The listing builds one solid part. Answer for the finished solid, in the listing's coordinates (mm). Give positions to 0.01 mm unless a question says otherwise; leave off trailing zeros. Write each loop counter-clockwise with the first axis right and the second up, starting at its lowest first coordinate (ties: lowest second). Pieces come first, ordered by that corner, then holes.
Autodesk Inventor part; units mm, degrees
ref_plane "YZ Plane" through (0, 0, 0) normal (1, 0, 0) x (0, 1, 0)
ref_plane "XZ Plane" through (0, 0, 0) normal (0, 1, 0) x (-1, 0, 0)
ref_plane "XY Plane" through (0, 0, 0) normal (0, 0, 1) x (1, 0, 0)
sketch "Sketch4" plane through (0, 0, 0) normal (1, 0, 0) x (0, 1, 0)
  line L0 (0, 0) -> (0, -26.0096)
  line L1 (0, 0) -> (33.46, 0)
  line L2 (33.46, 0) -> (33.46, -26.0096)
  line L3 (33.46, -26.0096) -> (0, -26.0096)
  line L4 (35.286, -25.908) -> (35.1766, -0.1801)
  arc A0 (35.286, -25.908) -> (35.2799, -24.4856) centre (35.283, -25.1968) ccw
  arc A1 (35.2795, -24.384) -> (35.2735, -22.9616) centre (35.2765, -23.6728) ccw
  arc A2 (35.273, -22.86) -> (35.267, -21.4376) centre (35.27, -22.1488) ccw
  arc A3 (35.2665, -21.336) -> (35.2605, -19.9137) centre (35.2635, -20.6248) ccw
  arc A4 (35.2601, -19.8121) -> (35.254, -18.3897) centre (35.257, -19.1009) ccw
  arc A5 (35.2536, -18.2881) -> (35.2475, -16.8657) centre (35.2506, -17.5769) ccw
  arc A6 (35.2471, -16.7641) -> (35.2411, -15.3417) centre (35.2441, -16.0529) ccw
  arc A7 (35.2406, -15.2401) -> (35.2346, -13.8177) centre (35.2376, -14.5289) ccw
  arc A8 (35.2342, -13.7161) -> (35.2281, -12.2937) centre (35.2311, -13.0049) ccw
  arc A9 (35.2277, -12.1921) -> (35.2216, -10.7697) centre (35.2247, -11.4809) ccw
  arc A10 (35.2212, -10.6681) -> (35.2152, -9.2458) centre (35.2182, -9.9569) ccw
  arc A11 (35.2147, -9.1442) -> (35.2087, -7.7218) centre (35.2117, -8.433) ccw
  arc A12 (35.2083, -7.6202) -> (35.2022, -6.1978) centre (35.2052, -6.909) ccw
  arc A13 (35.2018, -6.0962) -> (35.1957, -4.6738) centre (35.1988, -5.385) ccw
  arc A14 (35.1953, -4.5722) -> (35.1893, -3.1498) centre (35.1923, -3.861) ccw
  arc A15 (35.1888, -3.0482) -> (35.1828, -1.6258) centre (35.1858, -2.337) ccw
  arc A16 (35.1824, -1.5242) -> (35.1763, -0.1018) centre (35.1793, -0.813) ccw
  line L5 (35.1763, -0.1018) -> (33.46, -0.1018)
  line L6 (35.286, -25.908) -> (33.46, -25.908)
  point P0 (35.2799, -24.4856)
  point P1 (35.2735, -22.9616)
  point P2 (35.267, -21.4376)
  point P3 (35.2605, -19.9137)
  point P4 (35.254, -18.3897)
  point P5 (35.2536, -18.2881)
  point P6 (35.2475, -16.8657)
  point P7 (35.2411, -15.3417)
  point P8 (35.2406, -15.2401)
  point P9 (35.2346, -13.8177)
  point P10 (35.2342, -13.7161)
  point P11 (35.2281, -12.2937)
  point P12 (35.2277, -12.1921)
  point P13 (35.2216, -10.7697)
  point P14 (35.2152, -9.2458)
  point P15 (35.2087, -7.7218)
  point P16 (35.2083, -7.6202)
  point P17 (35.2022, -6.1978)
  point P18 (35.2018, -6.0962)
  point P19 (35.1957, -4.6738)
  point P20 (35.1953, -4.5722)
  point P21 (35.1893, -3.1498)
  point P22 (35.1888, -3.0482)
  point P23 (35.1828, -1.6258)
  point P24 (35.1824, -1.5242)
  dimension "d12" = 26.0096
  dimension "d13" = 33.46
  dimension "d14" = 1.8288
  dimension "d18" = 1.524
  dimension "d25" = 0.7112
  dimension "d26" = 0.243
  dimension "d27" = 0.1016
  dimension "d28" = 0
revolve "Revolution1" add sketch "Sketch4" angle 360 about axis through (0, 0, 0) along (0, 0, -1) contours L1 L2 L3 L0
sketch "Sketch5" plane through (0, 0, 0) normal (0, 0, 1) x (1, 0, 0)
  line L0 (19.05, 5.08) -> (19.05, -5.08)
  line L1 (28.575, 10.16) -> (28.575, -10.16)
  line L2 (28.575, 10.16) -> (19.05, 5.08)
  line L3 (19.05, -5.08) -> (28.575, -10.16)
  line L4 (5.4887, 29.8267) -> (5.1256, 19.0378)
  line L5 (5.4887, 29.8267) -> (23.0863, 19.6667)
  line L6 (5.1256, 19.0378) -> (13.9244, 13.9578)
  line L7 (13.9244, 13.9578) -> (23.0863, 19.6667)
  line L8 (-23.0863, 19.6667) -> (-13.9244, 13.9578)
  line L9 (-23.0863, 19.6667) -> (-5.4887, 29.8267)
  line L10 (-13.9244, 13.9578) -> (-5.1256, 19.0378)
  line L11 (-5.1256, 19.0378) -> (-5.4887, 29.8267)
  line L12 (-28.575, -10.16) -> (-19.05, -5.08)
  line L13 (-28.575, -10.16) -> (-28.575, 10.16)
  line L14 (-19.05, -5.08) -> (-19.05, 5.08)
  line L15 (-19.05, 5.08) -> (-28.575, 10.16)
  line L16 (-5.4887, -29.8267) -> (-5.1256, -19.0378)
  line L17 (-5.4887, -29.8267) -> (-23.0863, -19.6667)
  line L18 (-5.1256, -19.0378) -> (-13.9244, -13.9578)
  line L19 (-13.9244, -13.9578) -> (-23.0863, -19.6667)
  line L20 (23.0863, -19.6667) -> (13.9244, -13.9578)
  line L21 (23.0863, -19.6667) -> (5.4887, -29.8267)
  line L22 (13.9244, -13.9578) -> (5.1256, -19.0378)
  line L23 (5.1256, -19.0378) -> (5.4887, -29.8267)
  point P0 (0, 0)
  point P1 (19.05, 0)
  point P2 (28.575, 0)
  point P3 (14.2875, 24.7467)
  point P4 (9.525, 16.4978)
  point P5 (-14.2875, 24.7467)
  point P6 (-9.525, 16.4978)
  point P7 (-28.575, 0)
  point P8 (-19.05, 0)
  point P9 (-14.2875, -24.7467)
  point P10 (-9.525, -16.4978)
  point P11 (14.2875, -24.7467)
  point P12 (9.525, -16.4978)
  dimension "d30" = 10.16
  dimension "d31" = 20.32
  dimension "d32" = 0
  dimension "d33" = 19.05
  dimension "d34" = 9.525
  dimension "d35" = 0
  dimension "d38" = 360
extrude "Extrusion3" cut sketch "Sketch5" against normal through all
fillet "Fillet1" radius 2.54 24 edges at (-5.4887, -29.8267, -13.0048) (-5.1256, -19.0378, -13.0048) (-13.9244, -13.9578, -13.0048) (-23.0863, -19.6667, -13.0048) (5.4887, 29.8267, -13.0048) (5.1256, 19.0378, -13.0048) (13.9244, 13.9578, -13.0048) (23.0863, 19.6667, -13.0048) (-28.575, -10.16, -13.0048) (-19.05, -5.08, -13.0048) (-19.05, 5.08, -13.0048) (-28.575, 10.16, -13.0048) (23.0863, -19.6667, -13.0048) (13.9244, -13.9578, -13.0048) (5.1256, -19.0378, -13.0048) (5.4887, -29.8267, -13.0048) (28.575, 10.16, -13.0048) (19.05, 5.08, -13.0048) (19.05, -5.08, -13.0048) (28.575, -10.16, -13.0048) (-23.0863, 19.6667, -13.0048) (-13.9244, 13.9578, -13.0048) (-5.1256, 19.0378, -13.0048) (-5.4887, 29.8267, -13.0048)
sketch "Sketch6" plane through (0, 0, 0) normal (0, 0, 1) x (1, 0, 0)
  circle A0 centre (0, 0) radius 7.1
  circle A1 centre (-9.798, 5.6569) radius 2 construction
  circle A2 centre (5.6569, 9.798) radius 2 construction
  circle A3 centre (9.798, -5.6569) radius 2 construction
  circle A4 centre (-5.6569, -9.798) radius 2 construction
  circle A5 centre (-9.798, 5.6569) radius 2.15
  circle A6 centre (5.6569, 9.798) radius 2.15
  circle A7 centre (9.798, -5.6569) radius 2.15
  circle A8 centre (-5.6569, -9.798) radius 2.15
  dimension "d43" = 14.2
  dimension "d46" = 4.3
  dimension "d47" = 4.3
  dimension "d48" = 4.3
  dimension "d49" = 4.3
extrude "Extrusion4" cut sketch "Sketch6" against normal through all
properties part number "Wheel_Base"
Item 1: Consider probe 1 along X at (y, z) = (2, -21) (3 decimals); probe 2 along X at (y, z) = (1, -13) (3 decimals); probe 3 along X at (y, z) = (-20.5, -20). Determine where each line is inside the solid, lowest interval first.
Conclusion:
probe 1: x = -33.4 to -28.575, -19.05 to -6.812, 6.812 to 19.05, 28.575 to 33.4
probe 2: x = -33.445 to -28.575, -19.05 to -7.029, 7.029 to 19.05, 28.575 to 33.445
probe 3: x = -26.44 to -20.52, -5.18 to 5.18, 20.52 to 26.44
Item 2: A cutting plane is placed at B-B, the plane x = 0. Give the vertices of the cut face in (y, z).
Conclusion:
outline: (-33.46, -26.01) - (-7.1, -26.01) - (-7.1, 0) - (-33.46, 0) - close; (7.1, -26.01) - (33.46, -26.01) - (33.46, 0) - (7.1, 0) - close
Item 3: A cutting plane is placed at C-C, the plane x = 10.5. Give the vertices of the cut face in (y, z), plus the area to 3 significant figures.
Conclusion:
outline: (-31.77, -26.01) - (-26.93, -26.01) - (-26.93, 0) - (-31.77, 0) - close; (-15.93, -26.01) - (-7.69, -26.01) - (-7.69, 0) - (-15.93, 0) - close; (-3.62, -26.01) - (15.93, -26.01) - (15.93, 0) - (-3.62, 0) - close; (26.93, -26.01) - (31.77, -26.01) - (31.77, 0) - (26.93, 0) - close
area: 975 mm2
Item 4: Determine the mould class of faces 1 (the face through (-0.92, 7.04, -12.82)), 2 (the face through (-9.482, -16.523, -12.823)) for opening direction Y: pulls with the +Y half, pulls with the -Y half, needs draft (parallel to the pull), parting line crosses it, or undercut.
Conclusion:
face 1: undercut
face 2: undercut
Item 5: A cutting plane is placed at A-A, the plane y = 0. Give the vertices of the cut face in (x, z) (3 decimals).
Conclusion:
outline: (-33.46, -26.01) - (-28.575, -26.01) - (-28.575, 0) - (-33.46, 0) - close; (-19.05, -26.01) - (-7.1, -26.01) - (-7.1, 0) - (-19.05, 0) - close; (7.1, -26.01) - (19.05, -26.01) - (19.05, 0) - (7.1, 0) - close; (28.575, -26.01) - (33.46, -26.01) - (33.46, 0) - (28.575, 0) - close
Item 6: Each of these flat-tipped pins is pushed along its axis until it touches: P1, Ø6, axis at x = 13.5, z = -14.5, coming from the +Y side; P2, Ø2, axis at x = -15, z = -8, coming from the -Y side; P3, Ø2.5, axis at x = 9.8, y = -5.66, coming from the -Z side; P4, Ø8, axis at y = -1.5, z = -18.5, coming from the +X side. Where does it stop, or does it pass through?
Conclusion:
P1: stops at y = 31.77
P2: stops at y = -30.39
P3: passes through
P4: stops at x = 33.46
Item 7: A cutting plane is placed at D-D, the plane x = -17. Give the vertices of the cut face in (y, z), plus the area to 3 significant figures.
Conclusion:
outline: (-28.82, -26.01) - (-23.18, -26.01) - (-23.18, 0) - (-28.82, 0) - close; (-15.87, -26.01) - (15.87, -26.01) - (15.87, 0) - (-15.87, 0) - close; (23.18, -26.01) - (28.82, -26.01) - (28.82, 0) - (23.18, 0) - close
area: 1,120 mm2
